from build123d import *

# Parameters (mm, degrees)
SKETCH2_W               = 18.5
SKETCH2_H               = 25.41
BOSS_EXTRUDE1_DEPTH     = 9
CUT_EXTRUDE1_DEPTH      = 25.41
CUT_EXTRUDE3_DEPTH      = 33.694312961
CUT_EXTRUDE3_DEPTH_BACK = 25.41
SKETCH10_R              = 0.8
CUT_EXTRUDE4_DEPTH      = 33.694312961


with BuildPart() as part:
    # Sketch2 → Boss-Extrude1 (new body)
    with BuildSketch(Plane(origin=(0, 0, 0), x_dir=(1, 0, 0), z_dir=(0, 1, 0))):
        with Locations((9.25, 12.705)):
            Rectangle(SKETCH2_W, SKETCH2_H)
    extrude(amount=BOSS_EXTRUDE1_DEPTH)

    # Sketch6 → Cut-Extrude1 (cut)
    with BuildSketch(Plane.XY):
        with BuildLine():
            Line((2.9, 9), (15.6, 9))
            ThreePointArc((15.6, 9), (9.25, 2.65), (2.9, 9))
        make_face()
    extrude(amount=-CUT_EXTRUDE1_DEPTH, mode=Mode.SUBTRACT)

    # Sketch14 → Cut-Extrude3 (cut, two sides)
    with BuildSketch(Plane(origin=(0, 0, -25.41), x_dir=(-1, 0, 0), z_dir=(0, 0, -1))) as cut_extrude3_sk:
        Polygon((0, 60.146081223), (0, 9), (0, 7.5), (-3.246658661, 7.5), (-2.9, 9), (8.616604878, 58.832614185), (24.031387378, 159.956651774), (15.4147825, 161.270118812), align=None)
    extrude(amount=CUT_EXTRUDE3_DEPTH, mode=Mode.SUBTRACT)
    extrude(cut_extrude3_sk.sketch, amount=-CUT_EXTRUDE3_DEPTH_BACK, mode=Mode.SUBTRACT)


with BuildPart() as cut_extrude3_kept_piece:
    # of the separate pieces the step leaves, the one the design keeps (cut_extrude3_pieces_kept)
    add(part.part.solids().sort_by_distance((0, 0, 0))[0])

    # Sketch10 → Cut-Extrude4 (cut, through all)
    with BuildSketch(Plane(origin=(0, 9, 0), x_dir=(1, 0, 0), z_dir=(0, 1, 0))):
        with Locations(Location((17.05, 20.41, 0), (0, 0, 270))):
            Circle(SKETCH10_R)
        with Locations(Location((17.05, 5, 0), (0, 0, 270))):
            Circle(SKETCH10_R)
    extrude(amount=-CUT_EXTRUDE4_DEPTH, mode=Mode.SUBTRACT)


solid = cut_extrude3_kept_piece.part
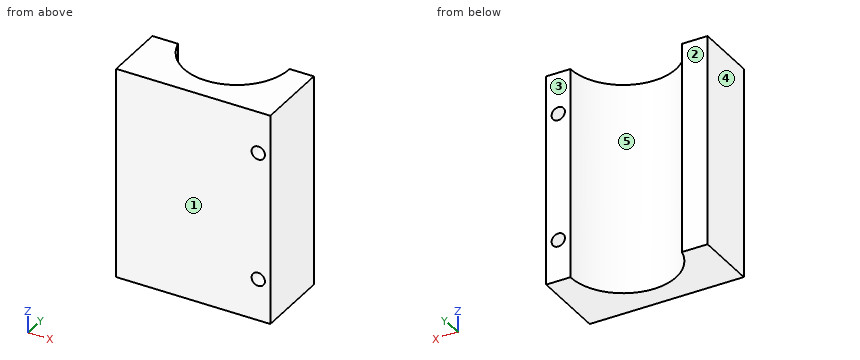
Can you work these out from the model? Positions are in its coordinate system, mm. Face numbers are marked on the shaded views. A direction names the side the tool comes from. Give positions to 0.01 mm unless a question says otherwise; leave off trailing zeros. Order: outer loops, then holes, each group sorted by start corner. A loop starts at its lowest first (then second) coordinate and runs counter-clockwise, first axis right, second up. Notation, with made-up numbers: M -20.5,-35.75 L -12.5,-35.75 A21 ccw -12.5,-2.75 Z; hole C 29.25,21 d9. An arc over 180 degrees is marked long. Use a Markdown table: item, result. Add a question column.
Item 1: Suppose I cut it at C-C (x = 17.05). List the corners of the cut face in (y, z) for me.
Item 2: Suppose I cut it at B-B (y = 3.25). List the corners of the cut face in (x, z) for me.
Item 3: Will this pin go through, and if not, where does the flat tip stop? pin 1 (2.5 mm diameter, centred on x = 2, z = -17, fed in from +Y).
Item 4: For the marked faces 1 and 2, which set-ups out of +Z, -Z, +X, -X, +Y, -Y let a thin tool reach every point of the face, with its end or its side?
Item 5: If I drill on L1, parallel to X at y = 6, z = -5; L2, parallel to X at y = 5, z = -20.41; L3, parallel to Y at x = 1.25, z = -18, over which ranges is the centre line in solid material (lowest first)? Write a range as [from, to].
Item 6: Suppose I cut it at D-D (y = 7). List the corners of the cut face in (x, z) for me.
Item 7: We'd pull the mould along X, two halves only. Please class the marked faces 3, 4 and 5: +X half, -X half, draft (parallel to the pull), parting line (faces both ways), or undercut.
Item 8: Suppose I cut it at A-A (z = -5). List the corners of the cut face in (x, y) for me, then the cut area to 3 significant figures.
Answer sheet:
| question | item | result |
|---|---|---|
| 1 | outline | M 0,-25.41 L 9,-25.41 L 9,-21.21 L 0,-21.21 Z; M 0,-19.61 L 9,-19.61 L 9,-5.8 L 0,-5.8 Z; M 0,-4.2 L 9,-4.2 L 9,0 L 0,0 Z |
| 2 | outline | M 0,-25.41 L 6.56,-25.41 L 6.56,0 L 0,0 Z; M 11.94,-25.41 L 18.5,-25.41 L 18.5,0 L 11.94,0 Z; hole C 17.05,-20.41 d1.6; hole C 17.05,-5 d1.6 |
| 3 | pin 1 | stops at y = 7.5 |
| 4 | face 1 | +Z, -Z, +X, -X, -Y |
| 4 | face 2 | +Z, -Z, -X, +Y |
| 5 | L1 | x = [0, 3.65], [14.85, 16.25], [17.85, 18.5] |
| 5 | L2 | x = [0, 4.32], [14.18, 16.25], [17.85, 18.5] |
| 5 | L3 | y = [0, 7.5] |
| 6 | outline | M 0,-25.41 L 3.22,-25.41 L 3.22,0 L 0,0 Z; M 15.28,-25.41 L 18.5,-25.41 L 18.5,0 L 15.28,0 Z; hole C 17.05,-20.41 d1.6; hole C 17.05,-5 d1.6 |
| 7 | face 3 | draft |
| 7 | face 4 | -X half |
| 7 | face 5 | undercut |
| 8 | outline | M 0,0 L 16.25,0 L 16.25,9 L 15.6,9 A6.35 cw 3.08,7.5 L 0,7.5 Z; M 17.85,0 L 18.5,0 L 18.5,9 L 17.85,9 Z |
| 8 | area | 84.3 mm² |
